```python
from build123d import *

# Parameters (mm, degrees)
SKETCH1_W           = 150
SKETCH1_H           = 150
BOSS_EXTRUDE1_DEPTH = 12.7
SKETCH2_W           = 10.53028371
SKETCH2_H           = 7.9375
SKETCH2_R           = 2.5
CUT_EXTRUDE1_DEPTH  = 12.7


with BuildPart() as part:
    # Sketch1 → Boss-Extrude1 (new body)
    with BuildSketch(Plane(origin=(0, 0, 0), x_dir=(1, 0, 0), z_dir=(0, 1, 0))):
        with Locations((75, 75)):
            Rectangle(SKETCH1_W, SKETCH1_H)
    extrude(amount=BOSS_EXTRUDE1_DEPTH)

    # Sketch2 → Cut-Extrude1 (cut)
    with BuildSketch(Plane(origin=(0, 12.7, 0), x_dir=(1, 0, 0), z_dir=(0, 1, 0))):
        with BuildLine():
            ThreePointArc((80.265141855, 82.9375), (83.392737967, 79.504173), (84.525, 75))
            Line((84.525, 75), (84.525, 90.875))
            Line((84.525, 90.875), (65.475, 90.875))
            Line((65.475, 90.875), (65.475, 75))
            ThreePointArc((65.475, 75), (66.607262033, 79.504173), (69.734858145, 82.9375))
            ThreePointArc((69.734858145, 82.9375), (75, 84.525), (80.265141855, 82.9375))
        make_face()
        with BuildLine():
            ThreePointArc((80.265141855, 67.0625), (83.392737967, 70.495827), (84.525, 75))
            Line((84.525, 75), (80.265141855, 75))
            Line((80.265141855, 75), (80.265141855, 67.0625))
        make_face()
        with BuildLine():
            Line((80.265141855, 75), (84.525, 75))
            ThreePointArc((84.525, 75), (83.392737967, 79.504173), (80.265141855, 82.9375))
            Line((80.265141855, 82.9375), (80.265141855, 75))
        make_face()
        with BuildLine():
            Line((69.734858145, 67.0625), (69.734858145, 75))
            Line((69.734858145, 75), (65.475, 75))
            ThreePointArc((65.475, 75), (66.607262033, 70.495827), (69.734858145, 67.0625))
        make_face()
        with BuildLine():
            Line((65.475, 75), (69.734858145, 75))
            Line((69.734858145, 75), (69.734858145, 82.9375))
            ThreePointArc((69.734858145, 82.9375), (66.607262033, 79.504173), (65.475, 75))
        make_face()
        with Locations((75, 78.96875)):
            Rectangle(SKETCH2_W, SKETCH2_H)
        with BuildLine():
            Line((69.734858145, 82.9375), (80.265141855, 82.9375))
            ThreePointArc((80.265141855, 82.9375), (75, 84.525), (69.734858145, 82.9375))
        make_face()
        with Locations((75, 71.03125)):
            Rectangle(SKETCH2_W, SKETCH2_H)
        with Locations((10, 140)):
            Circle(SKETCH2_R)
        with Locations((140, 140)):
            Circle(SKETCH2_R)
        with Locations((140, 10)):
            Circle(SKETCH2_R)
        with Locations((10, 10)):
            Circle(SKETCH2_R)
    extrude(amount=-CUT_EXTRUDE1_DEPTH, mode=Mode.SUBTRACT)


solid = part.part
```
Verification items for the finished model (mm, model axes). A direction names the side the tool comes from. Coordinates: 2 decimals unless noted, no trailing zeros. Loops run counter-clockwise (first coordinate to the right, second up) from the corner with the lowest first, then second, coordinate; pieces in that order, holes last. Notation, with made-up numbers: (70, 72.5) - (121, 72.5) arc R34 cw to (121, 104.5) - close; hole circle Ø9 at (36.5, 65). An arc over 180 degrees is marked (long way). Put each result on its own line as item: value.
Item 1: Scan lines: line 1 along Z through (x, y) = (140, 2.5); line 2 along X through (y, z) = (3.5, -140); line 3 along Z through (x, y) = (76, 1.75) (1 decimal). Record each from-to range of solid material in increasing order.
Conclusion:
line 1: z = -150 to -142.5, -137.5 to -12.5, -7.5 to 0
line 2: x = 0 to 7.5, 12.5 to 137.5, 142.5 to 150
line 3: z = -150 to -90.9, -67.1 to 0
Item 2: Section check C-C (z = -80). Enter the section's corners in (x, y) (3 decimals).
Conclusion:
outline: (0, 0) - (65.475, 0) - (65.475, 12.7) - (0, 12.7) - close; (84.525, 0) - (150, 0) - (150, 12.7) - (84.525, 12.7) - close
Item 3: Section check B-B (y = 6). Give the number of separate pieces and of enclosed holes in the cut face, then the cut area to 3 significant figures.
Conclusion:
separate pieces: 1
enclosed holes: 5
area: 22,000 mm2
Item 4: Section check A-A (x = 10). Enter the section's corners in (y, z).
Conclusion:
outline: (0, -150) - (12.7, -150) - (12.7, -142.5) - (0, -142.5) - close; (0, -137.5) - (12.7, -137.5) - (12.7, -12.5) - (0, -12.5) - close; (0, -7.5) - (12.7, -7.5) - (12.7, 0) - (0, 0) - close
Item 5: Section check D-D (z = -140). Enter the section's corners in (x, y).
Conclusion:
outline: (0, 0) - (7.5, 0) - (7.5, 12.7) - (0, 12.7) - close; (12.5, 0) - (137.5, 0) - (137.5, 12.7) - (12.5, 12.7) - close; (142.5, 0) - (150, 0) - (150, 12.7) - (142.5, 12.7) - close
Item 6: Gauge pin test, flat end, axial feed: pin 1 Ø6 at (x, z) = (140, -10) entering from +Y. Record the tip position at first contact, or that the pin passes through.
Conclusion:
pin 1: stops at y = 12.7
Item 7: Set-up check for faces 5 (the face through (65.475, 6, -83)), 6 (the face through (57, 0, -76)): record each of +Z, -Z, +X, -X, +Y, -Y from which the full face is reachable in a straight line by a thin tool's end or side.
Conclusion:
face 5: +Y, -Y
face 6: +Z, -Z, +X, -X, -Y
Item 8: Draft check along Z on faces 1 (the face through (57, 12.7, -76)), 2 (the face through (74, 6, -150)), 3 (the face through (66.58, 6.44, -70.55)), 4 (the face through (75, 6, -67.062)). Enter one of: pulls with the +Z half, pulls with the -Z half, needs draft (parallel to the pull), parting line crosses it, or undercut.
Conclusion:
face 1: needs draft
face 2: pulls with the -Z half
face 3: undercut
face 4: undercut
